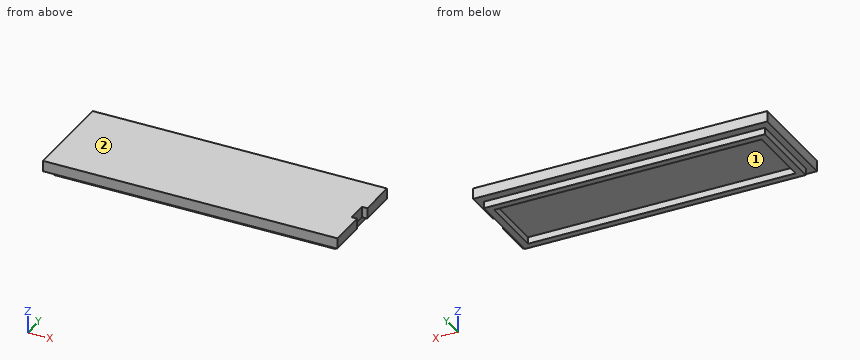
from build123d import *

# Parameters (mm, degrees)
F0_W     = 55.5
F0_H     = 18.3
F1_DEPTH = 2.032
F2_W     = 1.016
F2_H     = 3.81
F3_DEPTH = 2.286
F4_W     = 53
F4_H     = 15
F4_W_2   = 50.46
F4_H_2   = 12.46
F5_DEPTH = 1.27


with BuildPart() as f1:
    # F0 (on Top) → F1 (new body)
    with BuildSketch(Plane.XY):
        with Locations((18.105972, -2.473817)):
            Rectangle(F0_W, F0_H)
    extrude(amount=F1_DEPTH)

    # F2 (on face) → F3 (cut)
    with BuildSketch(Plane.XY.offset(2.032)):
        with Locations((45.347972, -2.473817)):
            Rectangle(F2_W, F2_H)
    extrude(amount=-F3_DEPTH, mode=Mode.SUBTRACT)

    # F4 (on face) → F5 (join)
    with BuildSketch(Plane(origin=(0, 0, 0), x_dir=(1, 0, 0), z_dir=(0, 0, -1))):
        with Locations((18.105972, 2.473817)):
            Rectangle(F4_W, F4_H)
        with Locations((18.105972, 2.473817)):
            Rectangle(F4_W_2, F4_H_2, mode=Mode.SUBTRACT)
    extrude(amount=F5_DEPTH)


solid = f1.part
Model file for the job. Use its own axes, mm. Face numbers are marked on the shaded views. Give positions to 0.01 mm unless a question says otherwise; leave off trailing zeros. Loops run counter-clockwise (first coordinate to the right, second up) from the corner with the lowest first, then second, coordinate; pieces in that order, holes last. Notation, with made-up numbers: (48, -5.75) -> (56, -5.75) arc R27 cw to (56, 23.25) -> close; hole circle Ø10 at (4, -38.5). An arc over 180 degrees is marked (long way). Use a Markdown table: item, result. Add a question column.
(1) Slice it at A-A on x = 13.5. List the corners of the cut face in (y, z), and give its area (3 significant figures).
(2) Slice it at B-B on y = 0.5. List the corners of the cut face in (x, z).
(3) Drop flat-ended pins along their axis: pin 1 Ø1.4 at (x, z) = (27, -1) entering from -Y; pin 2 Ø1.5 at (x, y) = (-1, 1) entering from -Z; pin 3 Ø0.6 at (x, z) = (8.5, -0.5) entering from +Y. Give the stop position or say it passes through.
(4) Mould opens along X. For the marked faces 1 and 2 say: +X half, -X half, draft (parallel to the pull), parting line (faces both ways), or undercut.
(5) Wall check: line 1 along Y through (x, z) = (11, -0.65); line 2 along Z through (x, y) = (9, 1); line 3 along X through (y, z) = (0, -0.1). Give the ranges that are in metal, low to high.
Filled sheet:
| question | item | result |
|---|---|---|
| 1 | outline | (-11.62, 0) -> (-9.97, 0) -> (-9.97, -1.27) -> (-8.7, -1.27) -> (-8.7, 0) -> (3.76, 0) -> (3.76, -1.27) -> (5.03, -1.27) -> (5.03, 0) -> (6.68, 0) -> (6.68, 2.03) -> (-11.62, 2.03) -> close |
| 1 | area | 40.4 mm2 |
| 2 | outline | (-9.64, 0) -> (-8.39, 0) -> (-8.39, -1.27) -> (-7.12, -1.27) -> (-7.12, 0) -> (43.34, 0) -> (43.34, -1.27) -> (44.61, -1.27) -> (44.61, 0) -> (45.86, 0) -> (45.86, 2.03) -> (-9.64, 2.03) -> close |
| 3 | pin 1 | y = -9.97 |
| 3 | pin 2 | z = 0 |
| 3 | pin 3 | y = 5.03 |
| 4 | face 1 | undercut |
| 4 | face 2 | draft |
| 5 | line 1 | -9.97 to -8.7, 3.76 to 5.03 |
| 5 | line 2 | 0 to 2.03 |
| 5 | line 3 | -8.39 to -7.12, 43.34 to 44.61 |
